from build123d import *

# Parameters (mm, degrees)
F0_W     = 110
F0_H     = 152.4
F0_R     = 3.56
F0_R_2   = 2.5
F1_DEPTH = 6.35
F2_R     = 5


# Not quite as in the source:
# - a length typed as a fraction of an inch, garbled in the dataset ("3 / 203.2 mm" for 3/8 in), is restored


with BuildPart() as f1:
    # F0 (on Top) → F1 (new body)
    with BuildSketch(Plane.XY):
        Rectangle(F0_W, F0_H)
        with Locations((-45.325, -64)):
            Circle(F0_R, mode=Mode.SUBTRACT)
        with Locations((-45.325, -45.325)):
            Circle(F0_R, mode=Mode.SUBTRACT)
        with Locations((45.325, -64)):
            Circle(F0_R_2, mode=Mode.SUBTRACT)
        with Locations((45.325, -45.325)):
            Circle(F0_R, mode=Mode.SUBTRACT)
        with Locations((11, -11)):
            Circle(F0_R_2, mode=Mode.SUBTRACT)
        with Locations((-11, 11)):
            Circle(F0_R_2, mode=Mode.SUBTRACT)
        with Locations((-45.325, 45.325)):
            Circle(F0_R_2, mode=Mode.SUBTRACT)
        with Locations((-45.325, 64)):
            Circle(F0_R, mode=Mode.SUBTRACT)
        with Locations((45.325, 45.325)):
            Circle(F0_R_2, mode=Mode.SUBTRACT)
        with Locations((45.325, 64)):
            Circle(F0_R_2, mode=Mode.SUBTRACT)
    extrude(amount=F1_DEPTH)

    # F2
    f2_edges = [f1.edges().sort_by_distance(p)[0] for p in [
        (-55, 76.2, 3.175),
        (55, 76.2, 3.175),
        (55, -76.2, 3.175),
        (-55, -76.2, 3.175),
    ]]
    fillet(f2_edges, radius=F2_R)


solid = f1.part
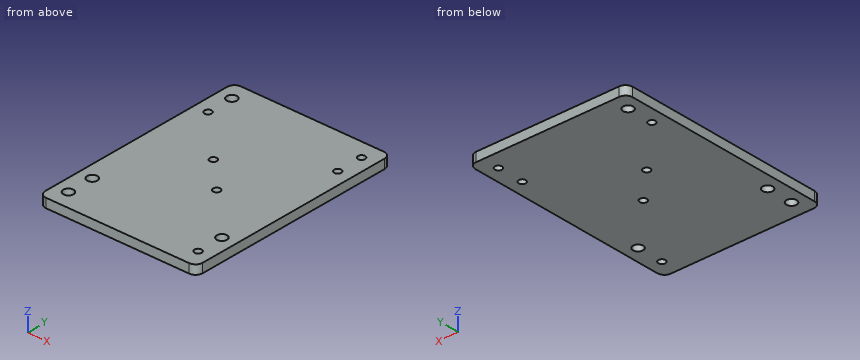
For this review, take the finished solid that the model builds, in its own axes (mm). Give positions to 0.01 mm unless a question says otherwise; leave off trailing zeros. Order: outer loops, then holes, each group sorted by start corner. A loop starts at its lowest first (then second) coordinate and runs counter-clockwise, first axis right, second up. Notation, with made-up numbers: M 68,53.5 L 94,53.5 A19 cw 94,59.5 Z; hole C 17,25.25 d8. An arc over 180 degrees is marked long. Answer in a Markdown table with one row per item. Add a question column.
(1) Consider section D-D on x = 11. State the section outline as (y, z) points, and give its area (3 significant figures).
(2) Wall thickness on probe 1 along X at (y, z) = (45.5, 2.25); probe 2 along X at (y, z) = (65, 6); probe 3 along Y at (x, z) = (-11, 3.75): over which ranges is each line inside the solid? List them lowest first. Write a range as [from, to].
(3) Consider section C-C on y = 64. State the section outline as (x, z) points (3 decimals).
(4) Consider section B-B on x = -46. State the section outline as (y, z) points, and give its area (3 significant figures).
(5) Consider section A-A on y = 11. State the section outline as (x, z) points.
Evaluation:
| question | item | result |
|---|---|---|
| 1 | outline | M -76.2,0 L -13.5,0 L -13.5,6.35 L -76.2,6.35 Z; M -8.5,0 L 76.2,0 L 76.2,6.35 L -8.5,6.35 Z |
| 1 | area | 936 mm^2 |
| 2 | probe 1 | x = [-55, -47.82], [-42.83, 42.83], [47.82, 55] |
| 2 | probe 2 | x = [-55, -48.74], [-41.91, 43.03], [47.62, 55] |
| 2 | probe 3 | y = [-76.2, 8.5], [13.5, 76.2] |
| 3 | outline | M -55,0 L -48.885,0 L -48.885,6.35 L -55,6.35 Z; M -41.765,0 L 42.825,0 L 42.825,6.35 L -41.765,6.35 Z; M 47.825,0 L 55,0 L 55,6.35 L 47.825,6.35 Z |
| 4 | outline | M -76.2,0 L -67.5,0 L -67.5,6.35 L -76.2,6.35 Z; M -60.5,0 L -48.82,0 L -48.82,6.35 L -60.5,6.35 Z; M -41.83,0 L 42.92,0 L 42.92,6.35 L -41.83,6.35 Z; M 47.73,0 L 60.5,0 L 60.5,6.35 L 47.73,6.35 Z; M 67.5,0 L 76.2,0 L 76.2,6.35 L 67.5,6.35 Z |
| 4 | area | 804 mm^2 |
| 5 | outline | M -55,0 L -13.5,0 L -13.5,6.35 L -55,6.35 Z; M -8.5,0 L 55,0 L 55,6.35 L -8.5,6.35 Z |
